Design review of the part shown in the three views and the two pictorial views. Dimensions are in mm from the part's minimum x, y and z. A direction names the side the tool comes from. Round coordinates to 2 decimals unless told otherwise and drop trailing zeros. Order: outer loops, then holes, each group sorted by start corner. A loop starts at its lowest first (then second) coordinate and runs counter-clockwise, first axis right, second up.
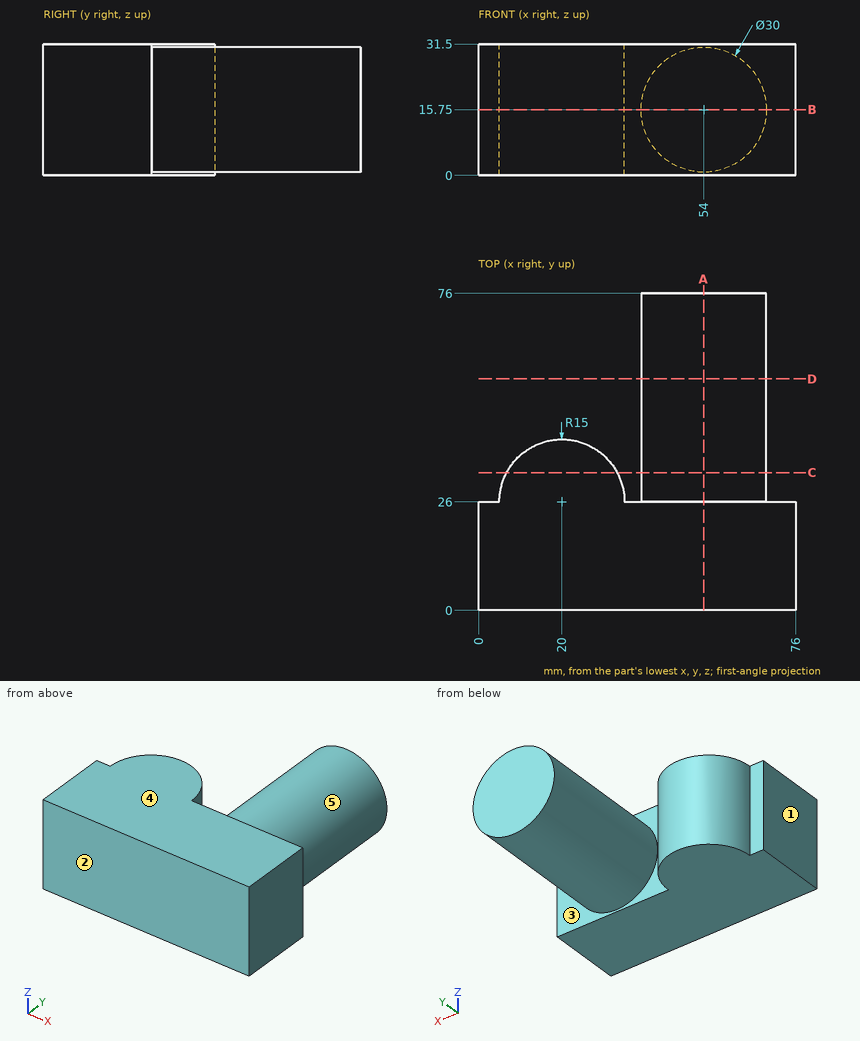
1) For the marked faces 4 and 5, list the 3-axis set-ups (+Z, -Z, +X, -X, +Y, -Y) from which the entire face can be reached by the end or side of a thin tool; tool diameter is ignored.
Results:
face 4: +Z, +X, -X, +Y, -Y
face 5: +Y
2) Take a section at C-C on y = 33. Give the boundary of the cut face in (x, z), plus the area to 3 significant figures.
Results:
outline: (6.73, 0) - (33.27, 0) - (33.27, 31.5) - (6.73, 31.5) - close; circle Ø30 at (54, 15.75)
area: 1,540 mm2
3) Clearance check with flat-ended pins moving along their axes: P1, Ø1.5, axis at x = 49.5, y = 28, coming from the -Z side; P2, Ø3, axis at y = 37, z = 26, coming from the +X side; P3, Ø2.5, axis at x = 3.5, z = 9.5, coming from the +Y side. State where each tip first meets the part, or that it passes through.
Results:
P1: stops at z = 1.23
P2: stops at x = 66.18
P3: stops at y = 26
4) The part is to be moulded in two halves that separate along X. For the marked faces 1, 2 and 3, say which applies: released by +X, released by -X, zero draft, split by the parting line, or undercut.
Results:
face 1: released by -X
face 2: zero draft
face 3: undercut
5) Take a section at D-D on y = 55.5. Give the boundary of the cut face in (x, z).
Results:
outline: circle Ø30 at (54, 15.75)
6) To check wall thickness, follow line 1 along X through (y, z) = (34.5, 9); line 2 along X through (y, z) = (46, 16.5); line 3 along X through (y, z) = (35.5, 23). State the ranges of each line that lie inside material, in increasing order.
Results:
line 1: x = 7.64 to 32.36, 40.6 to 67.4
line 2: x = 39.02 to 68.98
line 3: x = 8.39 to 31.61, 40.87 to 67.13
7) Take a section at B-B on z = 15.75. Give the boundary of the cut face in (x, y).
Results:
outline: (0, 0) - (76, 0) - (76, 26) - (69, 26) - (69, 76) - (39, 76) - (39, 26) - (35, 26) arc R15 ccw to (5, 26) - (0, 26) - close
8) Take a section at A-A on x = 54. Give the boundary of the cut face in (y, z).
Results:
outline: (0, 0) - (26, 0) - (26, 0.75) - (76, 0.75) - (76, 30.75) - (26, 30.75) - (26, 31.5) - (0, 31.5) - close
